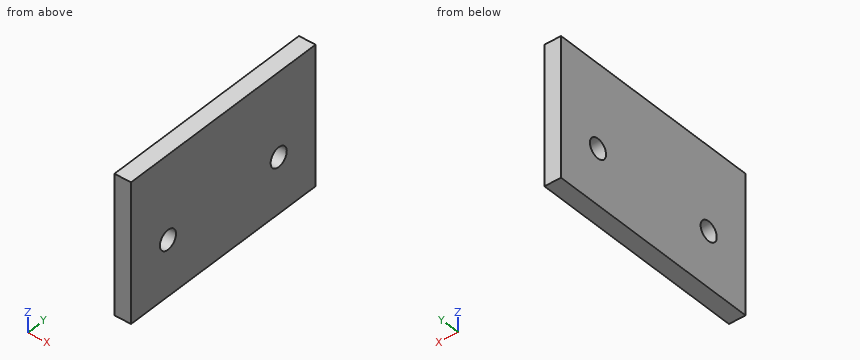
Autodesk Inventor part; units mm, degrees
ref_plane "Start Plane" through (0, 0, 0) normal (0, 0, 1) x (1, 0, 0)
ref_plane "End Plane" through (0, 0, 125) normal (0, 0, 1) x (1, 0, 0)
ref_plane "YZ Plane" through (0, 0, 0) normal (1, 0, 0) x (0, 1, 0)
ref_plane "Start Plane" through (0, 0, 0) normal (0, 0, 1) x (1, 0, 0)
ref_plane "End Plane" through (0, 0, 125) normal (0, 0, 1) x (1, 0, 0)
sketch "Sketch" plane through (0, 0, 0) normal (0, 0, 1) x (1, 0, 0)
  line L0 (7.5, -100) -> (-7.5, -100)
  line L1 (-7.5, -100) -> (-7.5, 100)
  line L2 (-7.5, 100) -> (7.5, 100)
  line L3 (7.5, 100) -> (7.5, -100)
  line L4 (-6, 0) -> (8, 0) construction
  line L5 (0, -30) -> (0, 40) construction
  line L6 (0, 140) -> (0, -140) construction
  line L7 (-11, 0) -> (13.5, 0) construction
  dimension "d0" = 200
  dimension "d1" = 15
  dimension "d4" = 7.5
  dimension "d5" = 100
extrude "Body" add sketch "Sketch" along normal up to surface (125 mm away) from surface at 0
sketch "Sketch3" plane through (0, 0, 0) normal (0, 0, 1) x (1, 0, 0)
  line L0 (0, 0) -> (10, 0)
ref_plane "Work Plane3" through (0, 0, 0) normal (0, -1, 0) x (1, 0, 0)
sketch "Sketch5" plane through (-7.5, 100, 0) normal (-1, 0, 0) x (0, 0, 1)
  point P0 (50, -40)
hole "Hole1" at (-7.5, 60, 50) direction (1, 0, 0) diameter 17.5 end through all
sketch "Sketch6" plane through (-7.5, 100, 0) normal (-1, 0, 0) x (0, 0, 1)
  point P0 (50, -160)
hole "Hole2" at (-7.5, -60, 50) direction (1, 0, 0) diameter 17.5 end through all
sketch "Sketch4" plane through (0, 0, 0) normal (0, -1, 0) x (1, 0, 0)
  line L0 (-2, 0) -> (12, 0)
  line L1 (-2, 125) -> (12, 125)
  dimension "d9" = 125
equation "\"d0\" = G_W"
equation "\"d1\" = G_H"
equation "\"d4\" = 0.5 * d1"
equation "\"d5\" = 0.5 * d0"
equation "\"d2\" = G_L"
equation "\"G_W\" = 200"
equation "\"G_H\" = 15"
equation "\"G_L\" = d9"
equation "\"G_OFFSET_START\" = 0"
equation "\"G_OFFSET_END\" = 0"
equation "\"d7\" = G_OFFSET_END + B_L"
equation "\"B_L\" = 125"
properties part number "DIN EN 10278 - 200 x 15 - 125" material "Steel, Mild"
Design review of the part built by this model. Coordinates are the model's own, in mm. Give positions to 0.01 mm unless a question says otherwise; leave off trailing zeros. Write each loop counter-clockwise with the first axis right and the second up, starting at its lowest first coordinate (ties: lowest second). Pieces come first, ordered by that corner, then holes.
(1) Add section C-C (x = 0.5). Give the boundary of the cut face in (y, z).
Checked values:
outline: (-100, 0) - (100, 0) - (100, 125) - (-100, 125) - close; hole circle Ø17.5 at (-60, 50); hole circle Ø17.5 at (60, 50)
(2) Add section A-A (z = 50). Give the boundary of the cut face in (x, y).
Checked values:
outline: (-7.5, -100) - (7.5, -100) - (7.5, -68.75) - (-7.5, -68.75) - close; (-7.5, -51.25) - (7.5, -51.25) - (7.5, 51.25) - (-7.5, 51.25) - close; (-7.5, 68.75) - (7.5, 68.75) - (7.5, 100) - (-7.5, 100) - close
(3) Wall thickness on line 1 along Y through (x, z) = (1.5, 50); line 2 along Z through (x, y) = (2.75, 60); line 3 along Z through (x, y) = (0.75, 64.5): over which ranges is each line inside the solid? List them lowest first.
Checked values:
line 1: y = -100 to -68.75, -51.25 to 51.25, 68.75 to 100
line 2: z = 0 to 41.25, 58.75 to 125
line 3: z = 0 to 42.5, 57.5 to 125
(4) Add section B-B (y = 60). Give the boundary of the cut face in (x, z), and give its area (3 significant figures).
Checked values:
outline: (-7.5, 0) - (7.5, 0) - (7.5, 41.25) - (-7.5, 41.25) - close; (-7.5, 58.75) - (7.5, 58.75) - (7.5, 125) - (-7.5, 125) - close
area: 1,610 mm2
